Geometry check sheet. Reference: the model listing, model coordinates, mm. A direction names the side the tool comes from. Give positions to 0.01 mm unless a question says otherwise; leave off trailing zeros. Loops run counter-clockwise (first coordinate to the right, second up) from the corner with the lowest first, then second, coordinate; pieces in that order, holes last. Notation, with made-up numbers: (83.5, -27) -> (110.5, -27) arc R22 cw to (110.5, 3) -> close; hole circle Ø5 at (52.5, 82.25). An arc over 180 degrees is marked (long way). Answer as a JSON object with one key per item and string values.
from build123d import *

# Parameters (mm, degrees)
SKETCH4_R           = 1.905
BOSS_EXTRUDE2_DEPTH = 50.8
SKETCH5_W           = 12.7
SKETCH5_H           = 8.89
CUT_EXTRUDE2_DEPTH  = 62.885856388
SKETCH6_R           = 3.175
CUT_EXTRUDE3_DEPTH  = 60.114292576


with BuildPart() as part:
    # Sketch4 → Boss-Extrude2 (new body)
    with BuildSketch(Plane(origin=(0, 0, 0), x_dir=(0, 0, -1), z_dir=(1, 0, 0))):
        with BuildLine():
            Line((29.794065187, -0.670981472), (4.394065187, -0.670981472))
            ThreePointArc((4.394065187, -0.670981472), (-4.137088067, 1.625585225), (3.675475152, -2.499781472))
            Line((3.675475152, -2.499781472), (29.794065187, -2.499781472))
            Line((29.794065187, -2.499781472), (29.794065187, -0.670981472))
        make_face()
        Circle(SKETCH4_R, mode=Mode.SUBTRACT)
    extrude(amount=BOSS_EXTRUDE2_DEPTH)

    # Sketch5 → Cut-Extrude2 (cut, through all)
    with BuildSketch(Plane(origin=(0, 14.569018528, 0), x_dir=(1, 0, 0), z_dir=(0, 1, 0))):
        with Locations((6.35, 0)):
            Rectangle(SKETCH5_W, SKETCH5_H)
        with Locations((31.75, 0)):
            Rectangle(SKETCH5_W, SKETCH5_H)
    extrude(amount=-CUT_EXTRUDE2_DEPTH, mode=Mode.SUBTRACT)

    # Sketch6 → Cut-Extrude3 (cut, through all)
    with BuildSketch(Plane(origin=(0, -0.670981472, 0), x_dir=(1, 0, 0), z_dir=(0, 1, 0))):
        with Locations(Location((12.663329801, 17.119532593, 0), (0, 0, 270))):
            Circle(SKETCH6_R)
        with Locations(Location((38.063329801, 17.119532593, 0), (0, 0, 270))):
            Circle(SKETCH6_R)
    extrude(amount=-CUT_EXTRUDE3_DEPTH, mode=Mode.SUBTRACT)


solid = part.part
1) Tool access check on faces 1 (the face through (38.1, -1, -2)), 2 (the face through (25, -2.5, -17)), 3 (the face through (0, -2, -17)), 4 (the face through (6, -2, -4.445)), 5 (the face through (44.36, -1.86, 0.41)). Record the directions out of +Z, -Z, +X, -X, +Y, -Y that give a thin tool (end or side, any length) a straight path to the whole face; none if there is none.
Geometry check:
{"face 1": "+Z, +Y, -Y", "face 2": "-Z, +X, -X, -Y", "face 3": "+Z, -Z, -X, +Y, -Y", "face 4": "+Z, -X, +Y, -Y", "face 5": "+X, -X"}
2) Section check A-A on y = 0. Record the cut outline in (x, z) (3 decimals).
Geometry check:
{"outline": "(12.7, -4.445) -> (25.4, -4.445) -> (25.4, -1.905) -> (12.7, -1.905) -> close; (12.7, 1.905) -> (25.4, 1.905) -> (25.4, 4.445) -> (12.7, 4.445) -> close; (38.1, -4.445) -> (50.8, -4.445) -> (50.8, -1.905) -> (38.1, -1.905) -> close; (38.1, 1.905) -> (50.8, 1.905) -> (50.8, 4.445) -> (38.1, 4.445) -> close"}
3) Depth check by flat-ended pin: P1, Ø6, axis at x = 34.5, z = -13.5, coming from the +Y side; P2, Ø4, axis at x = 32, y = 2, coming from the -Z side; P3, Ø4.5, axis at y = -0.5, z = -1, coming from the -X side; P4, Ø1, axis at x = 24, y = 1, coming from the -Z side. Enter the tip coordinate at first touch or a pass-through.
Geometry check:
{"P1": "stops at y = -0.67", "P2": "passes through", "P3": "stops at x = 12.7", "P4": "stops at z = -4.42"}
4) Draft check along Z on faces 6 (the face through (50.8, -1, -8)), 7 (the face through (18.96, -1.86, 0.41)), 8 (the face through (25, -2, -29.794)). Enter one of: pulls with the +Z half, pulls with the -Z half, needs draft (parallel to the pull), parting line crosses it, or undercut.
Geometry check:
{"face 6": "needs draft", "face 7": "undercut", "face 8": "pulls with the -Z half"}
5) Section check D-D on x = 16.5. Record the cut outline in (y, z) (3 decimals), plus the area to 3 significant figures.
Geometry check:
{"outline": "(-2.5, -29.794) -> (-0.671, -29.794) -> (-0.671, -4.394) arc R4.445 ccw (long way) to (-2.5, -3.675) -> close; hole circle Ø3.81 at (0, 0)", "area": "97.6 mm2"}
6) Material ranges on line 1 along X through (y, z) = (-1.75, 3); line 2 along Y through (x, z) = (41.25, 0) (3 decimals), recorded low to high. Write a range as from..to.
Geometry check:
{"line 1": "x = 12.7..25.4, 38.1..50.8", "line 2": "y = -4.445..-1.905, 1.905..4.445"}
7) Section check B-B on x = 39. Record the cut outline in (y, z) (3 decimals), plus the area to 3 significant figures.
Geometry check:
{"outline": "(-2.5, -29.794) -> (-0.671, -29.794) -> (-0.671, -20.153) -> (-2.5, -20.153) -> close; (-2.5, -14.086) -> (-0.671, -14.086) -> (-0.671, -4.394) arc R4.445 ccw (long way) to (-2.5, -3.675) -> close; hole circle Ø3.81 at (0, 0)", "area": "86.5 mm2"}
